```python
from build123d import *

# Parameters (mm, degrees)
F1_DEPTH = 25
F2_R     = 2
F3_DEPTH = 27
F4_SIZE  = 5


with BuildPart() as f1:
    # F0 (on Front) → F1 (new body)
    with BuildSketch(Plane.XZ):
        Polygon((-56, 134.6547987339), (-56, 69.6547987339), (-31, 69.6547987339), (-31, 109.6547987339), (0, 109.6547987339), (0, -155.3452012661), (0, -159.7533757838), (25, -155.3452012661), (182.569240482, -127.5614928394), (178.2939886904, -103.3153350796), (168.4459111603, -105.0518168562), (170.0087447593, -113.9150866333), (163.1150904882, -115.130623877), (161.5522568892, -106.2673540999), (25, -130.3452012661), (25, 134.6547987339), align=None)
    extrude(amount=F1_DEPTH)

    # F2 (on face) → F3 (cut)
    with BuildSketch(Plane(origin=(23.0441844496, 0, -130.6900643169), x_dir=(0.984807753, 0, 0.1736481777), z_dir=(-0.1736481777, 0, 0.984807753))):
        with Locations((62.6447827161, -12.5)):
            Circle(F2_R)
    extrude(amount=-F3_DEPTH, mode=Mode.SUBTRACT)

    # F4
    f4_edges = [f1.edges().sort_by_distance(p)[0] for p in [
        (25, -25, 2.154799),
        (25, 0, 2.154799),
        (-43.5, -25, 69.654799),
        (-56, -12.5, 69.654799),
        (-31, -12.5, 69.654799),
        (-43.5, 0, 69.654799),
    ]]
    chamfer(f4_edges, length=F4_SIZE)


solid = f1.part
```
The model under review builds one solid part; all positions refer to its coordinate system, in mm. A direction names the side the tool comes from. Round coordinates to 2 decimals unless told otherwise and drop trailing zeros. Loops run counter-clockwise (first coordinate to the right, second up) from the corner with the lowest first, then second, coordinate; pieces in that order, holes last. Notation, with made-up numbers: (-23.5, 65) -> (22.5, 65) arc R25 ccw to (22.5, 95) -> close; hole circle Ø10 at (-27, -25.5). An arc over 180 degrees is marked (long way). Answer as a JSON object with one key per item and string values. Group by question number.
1) We need section C-C on x = 65. Write out the cut boundary in (y, z).
2) We need section B-B on z = -73.5. Write out the cut boundary in (x, y).
3) For line 1 (X direction, y = -9.5, z = 75); line 2 (X direction, y = -6.75, z = 33.5); line 3 (X direction, y = -1.25, z = 74), list the stretches that pass through material, from the lowest coordinate up. Write a range as [from, to].
4) We need section A-A on z = 104.5. Write out the cut boundary in (x, y).
5) For pin 1 Ø1.5 at (x, y) = (27.5, -12.5) entering from +Z; pin 2 Ø8 at (x, y) = (94.5, -19.5) entering from +Z; pin 3 Ø4.5 at (y, z) = (-12, 31) entering from +X, all flat-tipped, find the tip position at first contact; note any pin that passes through.
6) For faces 4 (the face through (-16, -12, 109.655)), 5 (the face through (169.216, -12.325, -109.421)), 6 (the face through (162.345, -12.325, -110.761)), 7 (the face through (180.46, -12.32, -115.61)), list the 3-axis set-ups (+Z, -Z, +X, -X, +Y, -Y) from which the entire face can be reached by the end or side of a thin tool; tool diameter is ignored.
7) Mouldability with a two-part tool opening along Z and no side actions: class faces 1 (the face through (-44, -12, 69.655)), 2 (the face through (19, -25, -23)), 3 (the face through (166.61, -12.325, -114.514)) as released by +Z, released by -Z, zero draft, split by the parting line, or undercut.
Result set:
{
 "1": {"outline": "(-25, -148.29) -> (0, -148.29) -> (0, -123.29) -> (-25, -123.29) -> close"},
 "2": {"outline": "(0, -25) -> (20, -25) -> (25, -20) -> (25, -5) -> (20, 0) -> (0, 0) -> close"},
 "3": {"line 1": "[-56, -31], [0, 25]", "line 2": "[0, 25]", "line 3": "[-55.35, -31.65], [0, 21.25]"},
 "4": {"outline": "(-56, -25) -> (-31, -25) -> (-31, 0) -> (-56, 0) -> close; (0, -25) -> (20, -25) -> (25, -20) -> (25, -5) -> (20, 0) -> (0, 0) -> close"},
 "5": {"pin 1": "z = -129.77", "pin 2": "z = -117.39", "pin 3": "x = 25"},
 "6": {"face 4": "-Z, +Y, -Y", "face 5": "+Y, -Y", "face 6": "+Z, +Y, -Y", "face 7": "+Z, +X, +Y, -Y"},
 "7": {"face 1": "released by -Z", "face 2": "zero draft", "face 3": "undercut"}
}
